Source: CAD feature listing. Evaluate the final solid. Frame: model axes, mm. A direction names the side the tool comes from. Round coordinates to 2 decimals unless told otherwise and drop trailing zeros. Order: outer loops, then holes, each group sorted by start corner. A loop starts at its lowest first (then second) coordinate and runs counter-clockwise, first axis right, second up. Notation, with made-up numbers: (37, 69.5) -> (68, 69.5) arc R16 ccw to (68, 76.5) -> close; hole circle Ø8 at (70.5, -9.5). An arc over 180 degrees is marked (long way). One line per item, written item: value. Start each with the question number.
1) Section C-C (y = 12). State how many separate pieces and enclosed holes the cut face has, and give its area (3 significant figures).
2) Pin query (flat end, axial travel): P1, Ø8, axis at y = 16, z = -141, coming from the +X side; P2, Ø8, axis at x = -6, y = 17, coming from the -Z side; P3, Ø1.2, axis at x = -7.5, y = 8, coming from the -Z side; P4, Ø3, axis at x = -34, z = -131.5, coming from the -Y side. Return the tip coordinate at first contact, or that it passes through.
3) Reachability of faces 4 (the face through (-48.5, 15.33, -134.27)), 5 (the face through (20.9, 8.58, 8.25)), 6 (the face through (-6, 17.4, -8.5)), 7 (the face through (-33.642, 11.8, 6.4)) from +Z, -Z, +X, -X, +Y, -Y: full face, straight path, thin tool, end or side. Return the list, or none.
4) Section B-B (z = -142.5). Return the cut outline in (x, y).
5) Mould query, pull axis Y, two halves, no side actions, for faces 1 (the face through (-8, 12, -9.858)), 2 (the face through (-40, 24, -77)), 3 (the face through (-44.9, 12, -140)). Classes: pulls with the +Y half, pulls with the -Y half, needs draft (parallel to the pull), parting line crosses it, or undercut.
6) Section A-A (x = -20.5). Return the cut outline in (y, z), and give its area (3 significant figures).
7) Section D-D (z = -107). Return the cut outline in (x, y).
8) Ray query, L1, parallel to X at y = 8.5, z = -136.5; L2, parallel to X at y = 17.25, z = -108.5; L3, parallel to Z at x = -32.5, y = 11.25. Return the intervals inside material, ascending.
```python
from build123d import *

# Parameters (mm, degrees)
EXTRUDE_1_DEPTH          = 24
SKETCH_2_W               = 24
SKETCH_2_H               = 24
SKETCH_2_R               = 11.6
CUT_EXTRUDE_1_DEPTH      = 20
SKETCH_6_R               = 4.1
CUT_EXTRUDE_3_DEPTH      = 1
CUT_EXTRUDE_3_DEPTH_BACK = 67
FILLET_3_R               = 5
EXTRUDE_2_DEPTH          = 14
SKETCH_10_R              = 4.1
CUT_EXTRUDE_4_DEPTH      = 81
SKETCH_12_R              = 11.1
CUT_EXTRUDE_5_DEPTH      = 7.1
SKETCH_13_R              = 4.5
CUT_EXTRUDE_6_DEPTH      = 73.9


with BuildPart() as part:
    # Эскиз1 → Бобышка-Вытянуть1 (new body)
    with BuildSketch(Plane(origin=(0, 0, 0), x_dir=(1, 0, 0), z_dir=(0, 1, 0))):
        Polygon((-37.857864376, 37.857864376), (-36, 36), (-36, 159.857864376), (-52, 159.857864376), (-52, 23.715728753), align=None)
        Polygon((-36, 23.715728753), (-36, 36), (-37.857864376, 37.857864376), (-52, 23.715728753), align=None)
        Polygon((-33.642135624, 5.357864376), (-14.142135624, -14.142135624), (-14.142135624, 9.857864376), (-9.857864376, 9.857864376), (-36, 36), (-36, 23.715728753), (-52, 23.715728753), align=None)
        Polygon((-14.142135624, -14.142135624), (0, 0), (-9.857864376, 9.857864376), (-14.142135624, 9.857864376), align=None)
        Polygon((-9.857864376, 9.857864376), (0, 0), (-14.142135624, -14.142135624), (14, -14.142135624), (14, 9.857864376), align=None)
        Polygon((-33.642135624, -14.142135624), (-14.142135624, -14.142135624), (-33.642135624, 5.357864376), align=None)
    extrude(amount=EXTRUDE_1_DEPTH)

    # Эскиз2 → Вырез-Вытянуть1 (cut)
    with BuildSketch(Plane(origin=(14, 0, 0), x_dir=(0, 0, -1), z_dir=(1, 0, 0))):
        with Locations((-2.142135624, 12)):
            Rectangle(SKETCH_2_W, SKETCH_2_H)
        with Locations((-2.142135624, 12)):
            Circle(SKETCH_2_R, mode=Mode.SUBTRACT)
    extrude(amount=-CUT_EXTRUDE_1_DEPTH, mode=Mode.SUBTRACT)

    # Эскиз6 → Вырез-Вытянуть3 (cut, two sides)
    with BuildSketch(Plane(origin=(14, 0, 0), x_dir=(0, 0, -1), z_dir=(1, 0, 0))) as cut_extrude_3_sk:
        with Locations((-2.142135624, 12)):
            Circle(SKETCH_6_R)
    extrude(amount=CUT_EXTRUDE_3_DEPTH, mode=Mode.SUBTRACT)
    extrude(cut_extrude_3_sk.sketch, amount=-CUT_EXTRUDE_3_DEPTH_BACK, mode=Mode.SUBTRACT)

    # Скругление3
    fillet_3_edges = [part.edges().sort_by_distance(p)[0] for p in [
        (-19.821067812, 0, 14.142135624),
        (-19.821067812, 24, 14.142135624),
    ]]
    fillet(fillet_3_edges, radius=FILLET_3_R)

    # Эскиз9 → Бобышка-Вытянуть2 (add)
    with BuildSketch(Plane(origin=(14, 0, 0), x_dir=(0, 0, -1), z_dir=(1, 0, 0))):
        Polygon((0.420042203, 21.562177826), (-11.70431345, 14.562177826), (-4.70431345, 2.437822174), (7.420042203, 9.437822174), align=None)
    extrude(amount=EXTRUDE_2_DEPTH)

    # Эскиз10 → Вырез-Вытянуть4 (cut, through all)
    with BuildSketch(Plane(origin=(28, 0, 0), x_dir=(0, 0, -1), z_dir=(1, 0, 0))):
        with Locations((-2.142135624, 12)):
            Circle(SKETCH_10_R)
    extrude(amount=-CUT_EXTRUDE_4_DEPTH, mode=Mode.SUBTRACT)

    # Эскиз12 → Вырез-Вытянуть5 (cut)
    with BuildSketch(Plane.ZY.offset(52)):
        with Locations((-144.857864376, 12)):
            Circle(SKETCH_12_R)
    extrude(amount=-CUT_EXTRUDE_5_DEPTH, mode=Mode.SUBTRACT)

    # Эскиз13 → Вырез-Вытянуть6 (cut, through all)
    with BuildSketch(Plane.ZY.offset(44.9)):
        with Locations((-144.857864376, 12)):
            Circle(SKETCH_13_R)
    extrude(amount=-CUT_EXTRUDE_6_DEPTH, mode=Mode.SUBTRACT)


solid = part.part
```
Findings:
1. separate pieces: 3
1. enclosed holes: 0
1. area: 3,270 mm2
2. P1: x = -36
2. P2: z = -10
2. P3: z = -9.86
2. P4: through
3. face 4: -X
3. face 5: +Z, +X, -Y
3. face 6: +X
3. face 7: +Z, -X, +Y, -Y
4. outline: (-52, 0) -> (-36, 0) -> (-36, 8.17) -> (-44.9, 8.17) -> (-44.9, 1.15) -> (-52, 1.15) -> close; (-52, 22.85) -> (-44.9, 22.85) -> (-44.9, 15.83) -> (-36, 15.83) -> (-36, 24) -> (-52, 24) -> close
5. face 1: needs draft
5. face 2: pulls with the +Y half
5. face 3: undercut
6. outline: (0, -20.5) -> (24, -20.5) -> (24, 9.14) arc R5 ccw to (19, 14.14) -> (5, 14.14) arc R5 ccw to (0, 9.14) -> close; hole circle Ø8.2 at (12, 2.14)
6. area: 768 mm2
7. outline: (-52, 0) -> (-36, 0) -> (-36, 24) -> (-52, 24) -> close
8. L1: -44.9 to -36
8. L2: -52 to -36
8. L3: -32.5 to -1.89, 6.17 to 14.14
